```python
from build123d import *

# Parameters (mm, degrees)
BOSS_EXTRUDE1_DEPTH                                 = 3
FILLET1_R                                           = 2
CSK_FOR_M3_COUNTERSUNK_FLAT_HEAD_SCREW1_D           = 3.4
CSK_FOR_M3_COUNTERSUNK_FLAT_HEAD_SCREW1_CSINK_D     = 6.3
CSK_FOR_M3_COUNTERSUNK_FLAT_HEAD_SCREW1_CSINK_ANGLE = 90
FILLET2_R                                           = 0.25


with BuildPart() as part:
    # Sketch1 → Boss-Extrude1 (new, symmetric)
    with BuildSketch(Plane(origin=(0, 0, 0), x_dir=(1, 0, 0), z_dir=(0, 1, 0))):
        Polygon((-1.75, -9.875), (3.546572875, -9.875), (8.25, -5.171572875), (8.25, 5.171572875), (3.546572875, 9.875), (-1.75, 9.875), (-4.25, 7.875), (-7.25, 9.875), (-10.25, 6.875), (-10.25, 1), (-10.75, 1), (-10.75, -1), (-10.25, -1), (-10.25, -6.875), (-7.25, -9.875), (-4.25, -7.875), align=None)
        Polygon((-8.25, -6.875), (-8.25, 6.875), (-7.25, 7.875), (-5.25, 6.875), (-5.25, -6.875), (-7.25, -7.875), align=None, mode=Mode.SUBTRACT)
        Polygon((-3.25, -6.875), (-3.25, 6.875), (-2.25, 7.875), (-0.25, 6.875), (-0.25, -6.875), (-2.25, -7.875), align=None, mode=Mode.SUBTRACT)
    extrude(amount=BOSS_EXTRUDE1_DEPTH, both=True)

    # Fillet1
    fillet1_edges = [part.edges().sort_by_distance(p)[0] for p in [
        (3.546572875, 0, -9.875),
        (8.25, 0, -5.171572875),
        (8.25, 0, 5.171572875),
        (3.546572875, 0, 9.875),
    ]]
    fillet(fillet1_edges, radius=FILLET1_R)

    # CSK for M3 Countersunk Flat Head Screw1 (through all)
    with Locations(Plane(origin=(0, 3, 0), x_dir=(1, 0, 0), z_dir=(0, 1, 0))):
        with Locations((3.75, 4), (3.75, -4)):
            CounterSinkHole(CSK_FOR_M3_COUNTERSUNK_FLAT_HEAD_SCREW1_D / 2, CSK_FOR_M3_COUNTERSUNK_FLAT_HEAD_SCREW1_CSINK_D / 2, counter_sink_angle=CSK_FOR_M3_COUNTERSUNK_FLAT_HEAD_SCREW1_CSINK_ANGLE)

    # Fillet2
    fillet2_edges = [part.edges().sort_by_distance(p)[0] for p in [
        (-10.25, 0, -1),
        (-10.25, 0, 1),
    ]]
    fillet(fillet2_edges, radius=FILLET2_R)
    fillet2_2_edges = [part.edges().sort_by_distance(p)[0] for p in [
        (-10.75, 0, -1),
        (-10.75, 0, 1),
    ]]
    fillet(fillet2_2_edges, radius=FILLET2_R - 0.0001)  # a hair under: the kernel refuses the full size


solid = part.part
```
Can you work these out from the model? Positions are in its coordinate system, mm. A direction names the side the tool comes from. Round coordinates to 2 decimals unless told otherwise and drop trailing zeros. Loops run counter-clockwise (first coordinate to the right, second up) from the corner with the lowest first, then second, coordinate; pieces in that order, holes last. Notation, with made-up numbers: M -37,29.25 L 8,29.25 A33 ccw 8,57.25 Z; hole C 22.5,28.25 d7. An arc over 180 degrees is marked long. Answer as a JSON object with one key per item and string values. Group by question number.
Q1. Imagine slicing it at B-B, the plane x = 3.75. Please give me the cut outline in (y, z).
Q2. Imagine slicing it at A-A, the plane z = -4. Please give me the cut outline in (x, y).
Q3. Please list where these lines run through material, in increasing order: L1, parallel to X at y = -0.05, z = 4; L2, parallel to X at y = 0.3, z = -2.25; L3, parallel to X at y = -0.8, z = 0.5.
Q4. We'd pull the mould along Z, two halves only. Please class faces 4 (the flat face through (-2.757, 0.042, -7.368)), 5 (the flat face through (1, -3, 0)), 6 (the flat face through (1, 0, -9.875)): +Z half, -Z half, draft (parallel to the pull), parting line (faces both ways), or undercut.
Q5. Imagine slicing it at D-D, the plane y = 1.2. Count the separate pieces of the cut face and the enclosed holes in it, then the cut area to 3 significant figures.
Q6. On a 3-axis mill with a long thin cutter (end or side, diameter ignored), from which of +Z, -Z, +X, -X, +Y, -Y can I reach the whole of each face in a straight line? I mean faces 1 (the flat face through (-3.02, 0.04, 8.86)), 2 (the flat face through (-10.25, 0, 4)), 3 (the flat face through (-2.743, 0.042, 7.382)). Say none if no direction works.
Q7. Imagine slicing it at C-C, the plane x = -8. Please give me the cut outline in (y, z) (3 decimals), then the cut area to 3 significant figures.
Q8. Will these pins go through, and if not, where does the flat tip stop? pin 1 (4 mm diameter, centred on x = 3.75, z = -4, fed in from +Y); pin 2 (1 mm diameter, centred on y = -2, z = 6, fed in from -X); pin 3 (1 mm diameter, centred on x = -8.5, y = -1.5, fed in from +Z) (3 decimals).
Findings:
{
 "1": {"outline": "M -3,-9.59 L 3,-9.59 L 3,-7.15 L 1.55,-5.7 L -3,-5.7 Z; M -3,-2.3 L 1.55,-2.3 L 3,-0.85 L 3,0.85 L 1.55,2.3 L -3,2.3 Z; M -3,5.7 L 1.55,5.7 L 3,7.15 L 3,9.59 L -3,9.59 Z"},
 "2": {"outline": "M -10.25,-3 L -8.25,-3 L -8.25,3 L -10.25,3 Z; M -5.25,-3 L -3.25,-3 L -3.25,3 L -5.25,3 Z; M -0.25,-3 L 2.05,-3 L 2.05,1.55 L 0.6,3 L -0.25,3 Z; M 5.45,-3 L 8.25,-3 L 8.25,3 L 6.9,3 L 5.45,1.55 Z"},
 "3": {"L1": "x = -10.25 to -8.25, -5.25 to -3.25, -0.25 to 2.05, 5.45 to 8.25", "L2": "x = -10.25 to -8.25, -5.25 to -3.25, -0.25 to 8.25", "L3": "x = -10.75 to -8.25, -5.25 to -3.25, -0.25 to 8.25"},
 "4": {"face 4": "undercut", "face 5": "draft", "face 6": "-Z half"},
 "5": {"separate pieces": "1", "enclosed holes": "4", "area": "217 mm2"},
 "6": {"face 1": "+Z, +Y, -Y", "face 2": "+Z, -X, +Y, -Y", "face 3": "+Y, -Y"},
 "7": {"outline": "M -3,-9.125 L 3,-9.125 L 3,-7.125 L -3,-7.125 Z; M -3,7.125 L 3,7.125 L 3,9.125 L -3,9.125 Z", "area": "24.0 mm2"},
 "8": {"pin 1": "stops at y = 1.85", "pin 2": "stops at x = -10.25", "pin 3": "stops at z = 9.125"}
}
